Read the model definition and answer for the solid it produces. Units are mm, in the model's axes. Round coordinates to 2 decimals unless told otherwise and drop trailing zeros. Write each loop counter-clockwise with the first axis right and the second up, starting at its lowest first coordinate (ties: lowest second). Pieces come first, ordered by that corner, then holes. Notation, with made-up numbers: (42.5, 73) - (60.5, 73) arc R18 ccw to (60.5, 97) - close; hole circle Ø11 at (-27, 83.25). An arc over 180 degrees is marked (long way). One line per item, written item: value. Start each with the question number.
(1) A cutting plane is placed at A-A, the plane z = -38.1. Determine the outline of the cut face in (x, y) (3 decimals).
(2) A flat-ended cylindrical pin translates along its axis: pin 1 Ø3 at (x, z) = (-0.38, -25.4) entering from +Y. Find the tip coordinate at first contact, or state that the pin passes through.
(3) A cutting plane is placed at B-B, the plane y = 0.9. State how many separate pieces and enclosed holes the cut face has, plus the area to 3 significant figures.
(4) Find the intervals of material crossed by L1, parallel to Z at x = -13, y = 1.35; L2, parallel to X at y = 0.45, z = -38.5; L3, parallel to Z at x = -14.5, y = 1.3, in increasing order.
Autodesk Inventor part; units mm, degrees
ref_plane "YZ Plane" through (0, 0, 0) normal (1, 0, 0) x (0, 1, 0)
ref_plane "XZ Plane" through (0, 0, 0) normal (0, 1, 0) x (-1, 0, 0)
ref_plane "XY Plane" through (0, 0, 0) normal (0, 0, 1) x (1, 0, 0)
sketch "Sketch1" plane through (0, 0, 0) normal (0, 1, 0) x (-1, 0, 0)
  circle A0 centre (13.0821, 0) radius 2.4892
  circle A1 centre (0.3821, 0) radius 2.4892
  line L0 (0, 10.7252) -> (0, 9.1262) construction
  circle A2 centre (-12.3179, 0) radius 2.4892
  circle A3 centre (13.0821, -12.7) radius 2.4892
  circle A4 centre (0.3821, -12.7) radius 2.4892
  circle A5 centre (-12.3179, -12.7) radius 2.4892
  circle A6 centre (13.0821, -25.4) radius 2.4892
  circle A7 centre (0.3821, -25.4) radius 2.4892
  circle A8 centre (-12.3179, -25.4) radius 2.4892
  circle A9 centre (13.0821, -38.1) radius 2.4892
  circle A10 centre (0.3821, -38.1) radius 2.4892
  circle A11 centre (-12.3179, -38.1) radius 2.4892
  circle A12 centre (13.0821, -50.8) radius 2.4892
  circle A13 centre (0.3821, -50.8) radius 2.4892
  circle A14 centre (-12.3179, -50.8) radius 2.4892
  line L1 (21.7943, 12.7) -> (-21.0301, 12.7)
  line L2 (-25.0179, 8.7122) -> (-25.0179, -59.5122)
  line L3 (-21.0301, -63.5) -> (21.7943, -63.5)
  line L4 (25.7821, -59.5122) -> (25.7821, 8.7122)
  arc A15 (25.7821, 8.7122) -> (21.7943, 12.7) centre (21.7943, 8.7122) ccw
  arc A16 (-21.0301, 12.7) -> (-25.0179, 8.7122) centre (-21.0301, 8.7122) ccw
  arc A17 (-25.0179, -59.5122) -> (-21.0301, -63.5) centre (-21.0301, -59.5122) ccw
  arc A18 (21.7943, -63.5) -> (25.7821, -59.5122) centre (21.7943, -59.5122) ccw
  point P0 (0, 0)
  point P1 (-25.0179, -63.5)
  point P2 (-25.0179, 12.7)
  point P3 (25.7821, -63.5)
  dimension "d0" = 4.9784
  dimension "d1" = 4.9784
  dimension "d2" = 12.7
  dimension "d3" = 4.9784
  dimension "d4" = 12.7
  dimension "d7" = 12.7
  dimension "d14" = 50.8
  dimension "d15" = 76.2
  dimension "d16" = 3.9878
extrude "Extrusion1" add sketch "Sketch1" along normal blind 3.175
properties part number "3x5-Grid-Gusset"
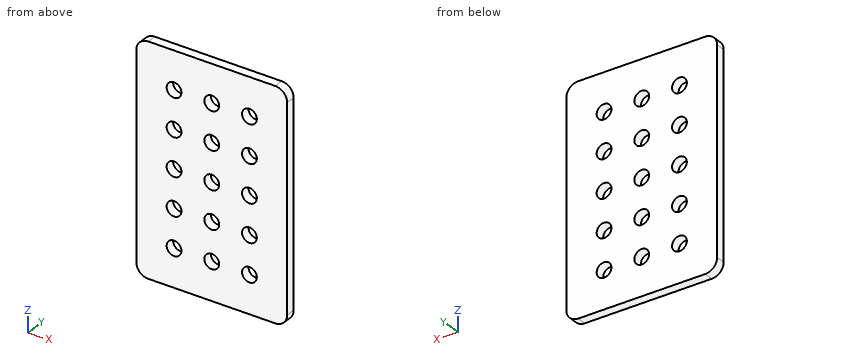
Here are the results:
1. outline: (-25.782, 0) - (-15.571, 0) - (-15.571, 3.175) - (-25.782, 3.175) - close; (-10.593, 0) - (-2.871, 0) - (-2.871, 3.175) - (-10.593, 3.175) - close; (2.107, 0) - (9.829, 0) - (9.829, 3.175) - (2.107, 3.175) - close; (14.807, 0) - (25.018, 0) - (25.018, 3.175) - (14.807, 3.175) - close
2. pin 1: through
3. separate pieces: 1
3. enclosed holes: 15
3. area: 3,570 mm²
4. L1: -63.5 to -53.29, -48.31 to -40.59, -35.61 to -27.89, -22.91 to -15.19, -10.21 to -2.49, 2.49 to 12.7
4. L2: -25.78 to -15.54, -10.63 to -2.84, 2.07 to 9.86, 14.77 to 25.02
4. L3: -63.5 to -52.85, -48.75 to -40.15, -36.05 to -27.45, -23.35 to -14.75, -10.65 to -2.05, 2.05 to 12.7
